Read the model definition and answer for the solid it produces. Units are mm, in the model's axes. Face numbers are marked on the shaded views. A direction names the side the tool comes from. Give positions to 0.01 mm unless a question says otherwise; leave off trailing zeros. Order: outer loops, then holes, each group sorted by start corner. A loop starts at its lowest first (then second) coordinate and runs counter-clockwise, first axis right, second up. Notation, with made-up numbers: (2.5, -24) - (11.5, -24) arc R22 cw to (11.5, -8) - close; hole circle Ø7 at (59, 67.25). An arc over 180 degrees is marked (long way). Write each question's results on one line, items separated by ' | '.
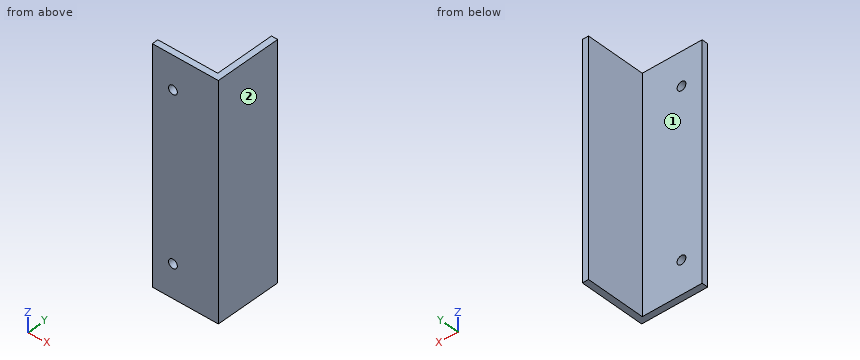
Autodesk Inventor part; units mm, degrees
ref_plane "YZ Plane" through (0, 0, 0) normal (1, 0, 0) x (0, 1, 0)
ref_plane "XZ Plane" through (0, 0, 0) normal (0, 1, 0) x (-1, 0, 0)
ref_plane "XY Plane" through (0, 0, 0) normal (0, 0, 1) x (1, 0, 0)
sketch "Sketch1" plane through (0, 0, 0) normal (0, 0, 1) x (1, 0, 0)
  line L0 (0, 50.8) -> (0, 0)
  line L1 (0, 0) -> (-50.8, 0)
  line L2 (-50.8, 0) -> (-50.8, 4.7752)
  line L3 (-50.8, 4.7752) -> (-4.7752, 4.7752)
  line L4 (-4.7752, 4.7752) -> (-4.7752, 50.8)
  line L5 (-4.7752, 50.8) -> (0, 50.8)
  dimension "d0" = 50.8
  dimension "d1" = 4.7752
extrude "Extrusion1" add sketch "Sketch1" along normal blind 177.8
hole "Hole1" at (-34.925, 4.7752, 25.4) direction (0, -1, 0) diameter 6.731 depth 25.4 tip angle 118
hole "Hole2" at (-34.925, 4.7752, 152.4) direction (0, -1, 0) diameter 6.731 depth 25.4 tip angle 118
properties part number "GE-12016-07"
(1) Each of these flat-tipped pins is pushed along its axis until it touches: pin 1 (23 mm diameter, centred on x = -21, z = 120, fed in from +Y); pin 2 (3 mm diameter, centred on y = 43.5, z = 44.5, fed in from +X); pin 3 (1 mm diameter, centred on y = 33, z = 134.5, fed in from -X); pin 4 (6 mm diameter, centred on x = -34.925, z = 152.4, fed in from -Y). Where does it stop, or does it pass through?
Conclusion:
pin 1: y = 4.78 | pin 2: x = 0 | pin 3: x = -4.78 | pin 4: through
(2) Section B-B (z = 13) is taken. Give the vertices of the cut face in (x, y), plus the area to 3 significant figures.
Conclusion:
outline: (-50.8, 0) - (0, 0) - (0, 50.8) - (-4.78, 50.8) - (-4.78, 4.78) - (-50.8, 4.78) - close | area: 462 mm^2
(3) Section C-C (y = 41) is taken. Give the vertices of the cut face in (x, z), plus the area to 3 significant figures.
Conclusion:
outline: (-4.78, 0) - (0, 0) - (0, 177.8) - (-4.78, 177.8) - close | area: 849 mm^2
(4) Consider probe 1 along X at (y, z) = (1, 152.4); probe 2 along X at (y, z) = (19, 117.5); probe 3 along Y at (x, z) = (-8.5, 132). Determine where each line is inside the solid, lowest interval first. Write a range as [from, to].
Conclusion:
probe 1: [-50.8, -38.29], [-31.56, 0] | probe 2: [-4.78, 0] | probe 3: [0, 4.78]
(5) Section A-A (z = 152.4) is taken. Give the vertices of the cut face in (x, y), plus the area to 3 significant figures.
Conclusion:
outline: (-50.8, 0) - (-38.29, 0) - (-38.29, 4.78) - (-50.8, 4.78) - close; (-31.56, 0) - (0, 0) - (0, 50.8) - (-4.78, 50.8) - (-4.78, 4.78) - (-31.56, 4.78) - close | area: 430 mm^2
(6) For the marked faces 1 and 2, determine the directions among +Z, -Z, +X, -X, +Y, -Y from which every point of the face is accessible in a straight line to the end or side of a thin tool.
Conclusion:
face 1: +Z, -Z, -X, +Y | face 2: +Z, -Z, +X, +Y, -Y
(7) Section D-D (x = -9.5) is taken. Give the vertices of the cut face in (y, z), plus the area to 3 significant figures.
Conclusion:
outline: (0, 0) - (4.78, 0) - (4.78, 177.8) - (0, 177.8) - close | area: 849 mm^2
